Read the model definition and answer for the solid it produces. Units are mm, in the model's axes. Give positions to 0.01 mm unless a question says otherwise; leave off trailing zeros. Write each loop counter-clockwise with the first axis right and the second up, starting at its lowest first coordinate (ties: lowest second). Pieces come first, ordered by that corner, then holes.
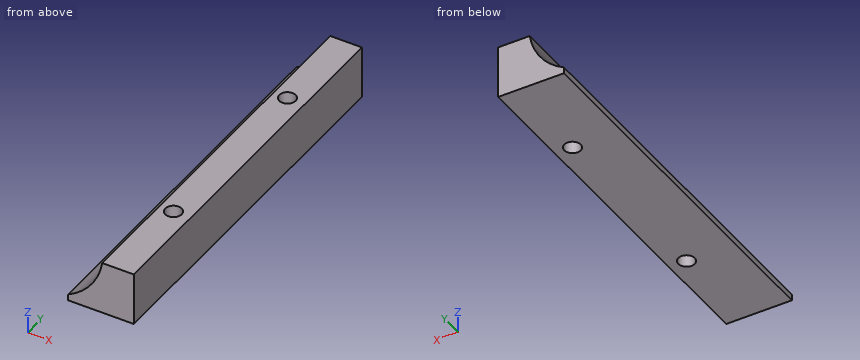
```python
from build123d import *

# Parameters (mm, degrees)
BOSS_EXTRUDE1_DEPTH        = 60
F_2_6_2_6_DIAMETER_HOLE1_D = 2.6


with BuildPart() as part:
    # Sketch1 → Boss-Extrude1 (new body)
    with BuildSketch(Plane(origin=(0, 0, 0), x_dir=(1, 0, 0), z_dir=(0, 1, 0))):
        with BuildLine():
            Line((0, 0), (0, 8.4))
            Line((0, 8.4), (-10.402546471, 8.4))
            Line((-10.402546471, 8.4), (-10.402546471, 7.4))
            ThreePointArc((-10.402546471, 7.4), (-6.785865437, 4.368315294), (-5, 0))
            Line((-5, 0), (0, 0))
        make_face()
    extrude(amount=BOSS_EXTRUDE1_DEPTH)

    # Ø2.6 (2.6) Diameter Hole1 (through all)
    with Locations(Plane(origin=(-2.75, 45, 0), x_dir=(1, 0, 0), z_dir=(0, 0, 1))):
        with Locations((0, 0), (0, -30)):
            Hole(F_2_6_2_6_DIAMETER_HOLE1_D / 2)


solid = part.part
```
Item 1: Section A-A (y = 15) is taken. Write down the section's boundary in (x, z) (3 decimals), and give its area (3 significant figures).
Result set:
outline: (-10.403, -8.4) - (-4.05, -8.4) - (-4.05, 0) - (-5, 0) arc R9.825 cw to (-10.403, -7.4) - close; (-1.45, -8.4) - (0, -8.4) - (0, 0) - (-1.45, 0) - close
area: 38.5 mm2
Item 2: Section D-D (y = 47) is taken. Write down the section's boundary in (x, z) (3 decimals), and give its area (3 significant figures).
Result set:
outline: (-10.403, -8.4) - (0, -8.4) - (0, 0) - (-5, 0) arc R9.825 cw to (-10.403, -7.4) - close
area: 60.4 mm2
Item 3: Section C-C (z = -4.75) is taken. Write down the section's boundary in (x, y), and give its area (3 significant figures).
Result set:
outline: (-7.08, 0) - (0, 0) - (0, 60) - (-7.08, 60) - close; hole circle Ø2.6 at (-2.75, 15); hole circle Ø2.6 at (-2.75, 45)
area: 414 mm2
Item 4: Section B-B (x = -2.75) is taken. Write down the section's boundary in (y, z).
Result set:
outline: (0, -8.4) - (13.7, -8.4) - (13.7, 0) - (0, 0) - close; (16.3, -8.4) - (43.7, -8.4) - (43.7, 0) - (16.3, 0) - close; (46.3, -8.4) - (60, -8.4) - (60, 0) - (46.3, 0) - close
Item 5: Find the intervals of material crossed by line 1 along Y through (x, z) = (-2.75, -5.5); line 2 along Z through (x, y) = (-6.5, 20.5); line 3 along Z through (x, y) = (-6, 6), in increasing order.
Result set:
line 1: y = 0 to 13.7, 16.3 to 43.7, 46.3 to 60
line 2: z = -8.4 to -3.95
line 3: z = -8.4 to -3.1
Item 6: This flat-tipped pin is pushed along its axis until it touches: pin 1 Ø4 at (x, z) = (-2, -1.5) entering from -Y. Where does it stop, or does it pass through?
Result set:
pin 1: stops at y = 0
